Build history of the part. All positions in model axes, mm. A direction names the side the tool comes from. Coordinates: 2 decimals unless noted, no trailing zeros. Loops run counter-clockwise (first coordinate to the right, second up) from the corner with the lowest first, then second, coordinate; pieces in that order, holes last. Notation, with made-up numbers: M 29,-3.5 L 72,-3.5 A18 ccw 72,27.5 Z; hole C 43,76.5 d4. An arc over 180 degrees is marked long. Write each question's results on one line, items separated by ' | '. Start each with the question number.
from build123d import *
from OCP.BRepFilletAPI import BRepFilletAPI_MakeFillet

# Parameters (mm, degrees)
SKETCH1_R              = 19.15
SKETCH1_R_2            = 6.35
BOSS_EXTRUDE1_DEPTH    = 3.175
F_10_CLEARANCE_HOLE1_D = 4.9784
FILLET1_R1             = 4
FILLET1_R2             = 10
CUT_EXTRUDE1_DEPTH     = 66.12085781
FILLET2_R              = 3.5


with BuildPart() as part:
    # Sketch1 → Boss-Extrude1 (new body)
    with BuildSketch(Plane.XY):
        with BuildLine():
            Line((54.139758885, 11.266432616), (22.225, 22.225))
            Line((22.225, 22.225), (-22.225, 22.225))
            Line((-22.225, 22.225), (-22.225, -22.225))
            Line((-22.225, -22.225), (22.225, -22.225))
            Line((22.225, -22.225), (54.905795434, -8.01403813))
            ThreePointArc((54.905795434, -8.01403813), (61.120351683, 1.888326902), (54.139758885, 11.266432616))
        make_face()
        Circle(SKETCH1_R, mode=Mode.SUBTRACT)
        with Locations((50.778511122, 1.477433)):
            Circle(SKETCH1_R_2, mode=Mode.SUBTRACT)
    extrude(amount=BOSS_EXTRUDE1_DEPTH)

    # 10 Clearance Hole1 (through all)
    with Locations(Plane.XY.offset(3.175)):
        with Locations((-17.960512242, 17.960512242), (17.960512242, 17.960512242), (17.960512242, -17.960512242), (-17.960512242, -17.960512242)):
            Hole(F_10_CLEARANCE_HOLE1_D / 2)

    # Fillet1: one fillet with a radius per group of edges: ONE call of the kernel's fillet builder (fillet() takes one radius for all edges)
    fillet1_edges_1 = [part.edges().sort_by_distance(p)[0] for p in [
        (-22.225, 22.225, 1.5875),
        (-22.225, -22.225, 1.5875),
    ]]
    fillet1_edges_2 = [part.edges().sort_by_distance(p)[0] for p in [
        (22.225, 22.225, 1.5875),
        (22.225, -22.225, 1.5875),
    ]]
    fillet1 = BRepFilletAPI_MakeFillet(part.part.solid().wrapped)
    for e in fillet1_edges_1:
        fillet1.Add(FILLET1_R1, e.wrapped)
    for e in fillet1_edges_2:
        fillet1.Add(FILLET1_R2, e.wrapped)
    add(Compound.cast(fillet1.Shape()), mode=Mode.REPLACE)

    # Sketch5 → Cut-Extrude1 (cut, through all)
    with BuildSketch(Plane.XY.offset(3.175)):
        with BuildLine():
            ThreePointArc((42.604398146, 7.82616335), (40.43667056, 1.066539098), (43.133854728, -5.499796294))
            Line((43.133854728, -5.499796294), (23.145734428, -14.191457916))
            ThreePointArc((23.145734428, -14.191457916), (27.148961622, 0.237450726), (22.893969402, 14.594131184))
            Line((22.893969402, 14.594131184), (42.604398146, 7.82616335))
        make_face()
    extrude(amount=-CUT_EXTRUDE1_DEPTH, mode=Mode.SUBTRACT)

    # Fillet2
    fillet2_edges = [part.edges().sort_by_distance(p)[0] for p in [
        (42.604398146, 7.82616335, 1.5875),
        (43.133854728, -5.499796294, 1.5875),
        (23.145734428, -14.191457916, 1.5875),
        (22.893969402, 14.594131184, 1.5875),
    ]]
    fillet(fillet2_edges, radius=FILLET2_R)


solid = part.part
1. Band-saw the part on C-C, the plane y = 0. Give the number of separate pieces and of enclosed holes in the cut face, plus the area to 3 significant figures.
2. Band-saw the part on B-B, the plane y = -14. List the corners of the cut face in (x, z) (3 decimals).
3. Band-saw the part on A-A, the plane x = 0. List the corners of the cut face in (y, z) (3 decimals).
4. Which spindle directions (+Z, -Z, +X, -X, +Y, -Y) get a long thin tool onto all of the face, cutting with end or side? Do faces 4 (the cylindrical face through (-21.022, 21.084, 1.61)), 5 (the flat face through (35.32, -8.898, 1.61)). Say none if no direction does.
5. Mould opens along Y. For faces 1 (the flat face through (19, 5, 0)), 2 (the flat face through (39.3, -14.8, 1.6)), 3 (the cylindrical face through (41.253, -5.243, 1.565)) say: +Y half, -Y half, draft (parallel to the pull), parting line (faces both ways), or undercut.
6. Pin check, flat tip, straight feed: pin 1 (1.5 mm diameter, centred on y = -7, z = 2.5, fed in from +X). Stop position of the tip, or through.
7. Wall check: line 1 along X through (y, z) = (-1.5, 2.85) (3 decimals); line 2 along X through (y, z) = (9, 1.75) (3 decimals); line 3 along X through (y, z) = (-3, 2.6) (3 decimals). Give the ranges that are in metal, low to high.
Checked values:
1) separate pieces: 4 | enclosed holes: 0 | area: 61.0 mm²
2) outline: M -22.225,0 L -13.066,0 L -13.066,3.175 L -22.225,3.175 Z; M 13.066,0 L 41.14,0 L 41.14,3.175 L 13.066,3.175 Z
3) outline: M -22.225,0 L -19.15,0 L -19.15,3.175 L -22.225,3.175 Z; M 19.15,0 L 22.225,0 L 22.225,3.175 L 19.15,3.175 Z
4) face 4: +Z, -Z, -X, +Y | face 5: +Z, -Z
5) face 1: draft | face 2: -Y half | face 3: undercut
6) pin 1: x = 57.66
7) line 1: -22.225 to -19.091, 19.091 to 27.109, 40.866 to 45.17, 56.387 to 60.691 | line 2: -22.225 to -16.903, 16.903 to 25.918, 39.122 to 57.887 | line 3: -22.225 to -18.914, 18.914 to 26.984, 41.399 to 46.276, 55.281 to 60.11
